from build123d import *

# Parameters (mm, degrees)
BOSS_EXTRUDE1_DEPTH = 10
SKETCH2_R           = 27
SKETCH2_R_2         = 3
BOSS_EXTRUDE2_DEPTH = 2.5


with BuildPart() as part:
    # Sketch1 → Boss-Extrude1 (new body)
    with BuildSketch(Plane(origin=(0, 0, 0), x_dir=(1, 0, 0), z_dir=(0, 1, 0))):
        with BuildLine():
            Line((-22.669793675, 8.750454545), (-14.273573795, 5.509545455))
            ThreePointArc((-14.273573795, 5.509545455), (0, 15.3), (14.273573795, 5.509545455))
            Line((14.273573795, 5.509545455), (22.669793675, 8.750454545))
            ThreePointArc((22.669793675, 8.750454545), (0, 24.3), (-22.669793675, 8.750454545))
        make_face()
    extrude(amount=BOSS_EXTRUDE1_DEPTH)

    # Sketch2 → Boss-Extrude2 (add)
    with BuildSketch(Plane.XZ):
        with Locations(Location((0, 0, 0), (0, 0, 270))):
            Circle(SKETCH2_R)
        with Locations(Location((0, 0, 0), (0, 0, 270))):
            Circle(SKETCH2_R_2, mode=Mode.SUBTRACT)
    extrude(amount=BOSS_EXTRUDE2_DEPTH)


solid = part.part
Build history of the part. All positions in model axes, mm. A direction names the side the tool comes from. Coordinates: 2 decimals unless noted, no trailing zeros. Order: outer loops, then holes, each group sorted by start corner. A loop starts at its lowest first (then second) coordinate and runs counter-clockwise, first axis right, second up. Notation, with made-up numbers: (30, 70) - (63, 70) arc R19 ccw to (63, 87) - close; hole circle Ø9 at (57, 39). An arc over 180 degrees is marked (long way). Write item = value, one per line. Start each with the question number.
1) Saw through at A-A on x = 0. Write the cut outline in (y, z).
2) Wall check: line 1 along X through (y, z) = (-1, 0); line 2 along Y through (x, z) = (-11.5, 3); line 3 along X through (y, z) = (4.75, -18). Give the ranges that are in metal, low to high. Write a range as from..to.
3) Saw through at D-D on x = -17.5. Write the cut outline in (y, z), then the cut area to 3 significant figures.
4) Two-plate mould, pull along X, no slides. Class faces 1 (the face through (18.413, 4.93, -7.107)), 2 (the face through (0.9, -1.23, -2.86)), 3 (the face through (0, 0, 6)), 4 (the face through (0, 10, -17)): pulls with the +X half, pulls with the -X half, needs draft (parallel to the pull), parting line crosses it, or undercut.
5) 3-axis set-ups, long thin cutter, end or side, ignore diameter. For faces 5 (the face through (0, -2.5, -6)), 6 (the face through (0.409, 4.93, -24.297)), 7 (the face through (-0.258, 4.93, -15.298)), 8 (the face through (-18.53, 4.93, -7.153)), 9 (the face through (-26.36, -1.23, 5.85)): which of +Z, -Z, +X, -X, +Y, -Y reach the whole face in a straight line?
6) Flat gauge pins, fed straight in: pin 1 Ø7 at (x, z) = (0, 0) entering from +Y; pin 2 Ø5 at (y, z) = (4.5, -16.5) entering from +X; pin 3 Ø6 at (y, z) = (1, 8.5) entering from -X. Where does each tip first touch, or does it go through?
7) Saw through at B-B on z = 0. Write the cut outline in (x, y).
8) Saw through at C-C on y = 6.25. Write the cut outline in (x, z).
From the geometry:
q1.outline = (-2.5, -27) - (0, -27) - (0, -24.3) - (10, -24.3) - (10, -15.3) - (0, -15.3) - (0, -3) - (-2.5, -3) - close; (-2.5, 3) - (0, 3) - (0, 27) - (-2.5, 27) - close
q2.line_1 = -27..-3, 3..27
q2.line_2 = -2.5..0
q2.line_3 = -16.32..16.32
q3.outline = (-2.5, -20.56) - (0, -20.56) - (0, -16.86) - (10, -16.86) - (10, -6.75) - (0, -6.75) - (0, 20.56) - (-2.5, 20.56) - close
q3.area = 204 mm^2
q4.face_1 = pulls with the +X half
q4.face_2 = undercut
q4.face_3 = undercut
q4.face_4 = needs draft
q5.face_5 = +Z, -Z, +X, -X, -Y
q5.face_6 = -Z, +Y
q5.face_7 = +Z, +Y
q5.face_8 = +Z, -X, +Y
q5.face_9 = +Y, -Y
q6.pin_1 = 0
q6.pin_2 = 19.86
q6.pin_3 = -26.4
q7.outline = (-27, -2.5) - (-3, -2.5) - (-3, 0) - (-27, 0) - close; (3, -2.5) - (27, -2.5) - (27, 0) - (3, 0) - close
q8.outline = (-22.67, -8.75) arc R24.3 ccw to (22.67, -8.75) - (14.27, -5.51) arc R15.3 cw to (-14.27, -5.51) - close
